from build123d import *

# Parameters (mm, degrees)
F1_DEPTH = 152.4
F3_D     = 9.525


with BuildPart() as f1:
    # F0 (on Front) → F1 (new body)
    with BuildSketch(Plane.XZ):
        Polygon((3.175, 25.4), (0, 25.4), (0, 0), (25.4, 0), (25.4, 3.175), (3.175, 3.175), align=None)
    extrude(amount=F1_DEPTH)

    # F3 (through all)
    with Locations(Plane(origin=(0, 0, 0), x_dir=(0, -1, 0), z_dir=(-1, 0, 0))):
        with Locations((44.45, 16.497891), (107.95, 16.497891)):
            Hole(F3_D / 2)


solid = f1.part
Work out the finished part from the listing and answer in its coordinate system (mm). A direction names the side the tool comes from. Give positions to 0.01 mm unless a question says otherwise; leave off trailing zeros. Loops run counter-clockwise (first coordinate to the right, second up) from the corner with the lowest first, then second, coordinate; pieces in that order, holes last. Notation, with made-up numbers: (53, -24.5) -> (98, -24.5) arc R5 cw to (98, -19.5) -> close; hole circle Ø5 at (1, 7). An arc over 180 degrees is marked (long way). Use a Markdown table: item, result. Add a question column.
1. Find the intervals of material crossed by probe 1 along Z at (x, y) = (2, -107.95); probe 2 along Y at (x, z) = (3, 15.5); probe 3 along Y at (x, z) = (1, 19.5), in increasing order.
2. For faces 5 (the flat face through (13, -75, 0)), 6 (the flat face through (3.175, -75, 14)), determine the directions among +Z, -Z, +X, -X, +Y, -Y from which every point of the face is accessible in a straight line to the end or side of a thin tool.
3. Section B-B on z = 15 is taken. Determine the outline of the cut face in (x, y) (3 decimals), and give its area (3 significant figures).
4. Section A-A on y = -44.45 is taken. Determine the outline of the cut face in (x, z) (3 decimals).
5. Determine the mould class of faces 1 (the cylindrical face through (1.61, -42.252, 12.273)), 2 (the flat face through (7, 0, 2)), 3 (the flat face through (2, -75, 25.4)), 4 (the flat face through (7, -152.4, 2)) for opening direction Y: released by +Y, released by -Y, zero draft, split by the parting line, or undercut.
6. Section D-D on x = 9.75 is taken. Determine the outline of the cut face in (y, z) (3 decimals).
7. Section C-C on y = -139.5 is taken. Determine the outline of the cut face in (x, z) (3 decimals).
8. Flat-ended cylindrical pins translate along their axes: pin 1 Ø1.5 at (x, y) = (15.5, -92.5) entering from +Z (3 decimals); pin 2 Ø12 at (y, z) = (-55, 11) entering from +X (3 decimals). Find the tip coordinate at first contact, or state that the pin passes through.
Results below:
| question | item | result |
|---|---|---|
| 1 | probe 1 | z = 0 to 11.74, 21.26 to 25.4 |
| 1 | probe 2 | y = -152.4 to -112.61, -103.29 to -49.11, -39.79 to 0 |
| 1 | probe 3 | y = -152.4 to -111.65, -104.25 to -48.15, -40.75 to 0 |
| 2 | face 5 | -Z, +X, -X, +Y, -Y |
| 2 | face 6 | +Z, +X, +Y, -Y |
| 3 | outline | (0, -152.4) -> (3.175, -152.4) -> (3.175, -112.471) -> (0, -112.471) -> close; (0, -103.429) -> (3.175, -103.429) -> (3.175, -48.971) -> (0, -48.971) -> close; (0, -39.929) -> (3.175, -39.929) -> (3.175, 0) -> (0, 0) -> close |
| 3 | area | 426 mm^2 |
| 4 | outline | (0, 0) -> (25.4, 0) -> (25.4, 3.175) -> (3.175, 3.175) -> (3.175, 11.735) -> (0, 11.735) -> close; (0, 21.26) -> (3.175, 21.26) -> (3.175, 25.4) -> (0, 25.4) -> close |
| 5 | face 1 | undercut |
| 5 | face 2 | released by +Y |
| 5 | face 3 | zero draft |
| 5 | face 4 | released by -Y |
| 6 | outline | (-152.4, 0) -> (0, 0) -> (0, 3.175) -> (-152.4, 3.175) -> close |
| 7 | outline | (0, 0) -> (25.4, 0) -> (25.4, 3.175) -> (3.175, 3.175) -> (3.175, 25.4) -> (0, 25.4) -> close |
| 8 | pin 1 | stops at z = 3.175 |
| 8 | pin 2 | stops at x = 3.175 |
